For this review, take the finished solid that the model builds, in its own axes (mm). Face numbers are marked on the shaded views. Round coordinates to 2 decimals unless told otherwise and drop trailing zeros. Write each loop counter-clockwise with the first axis right and the second up, starting at its lowest first coordinate (ties: lowest second). Pieces come first, ordered by that corner, then holes. Notation, with made-up numbers: M 6,23 L 20,23 A30 cw 20,56 Z; hole C 63,14.5 d7. An arc over 180 degrees is marked long. Answer in a Markdown table with one row per item.
```python
from build123d import *

# Parameters (mm, degrees)
F0_R     = 14.8209
F0_R_2   = 9.525
F1_DEPTH = 39.116
F2_SIZE2 = 1.524
F2_SIZE  = 1.524
F5_D     = 9.525


with BuildPart() as f1:
    # F0 (on Top) → F1 (new body)
    with BuildSketch(Plane.XY):
        Circle(F0_R)
        Circle(F0_R_2, mode=Mode.SUBTRACT)
    extrude(amount=F1_DEPTH)

    # F2
    f2_edges = [f1.edges().sort_by_distance(p)[0] for p in [
        (-14.8209, 0, 39.116),
    ]]
    chamfer(f2_edges, length=F2_SIZE, length2=F2_SIZE2)

    # F5 (through all)
    with Locations(Plane.XZ.offset(14.8209)):
        with Locations((0, 26.416)):
            Hole(F5_D / 2)


solid = f1.part
```
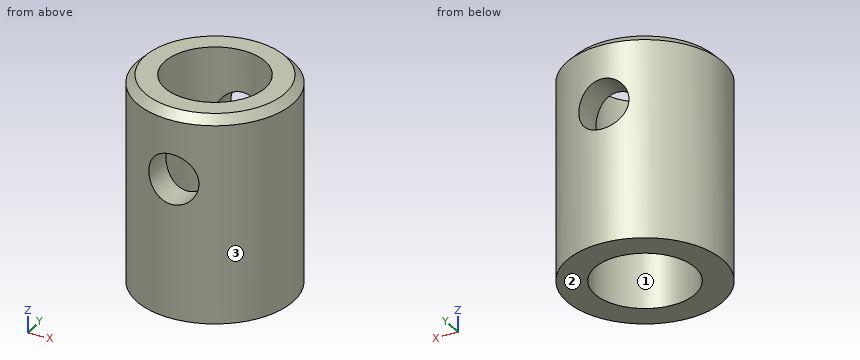
Q1. Take a section at D-D (z = 10). State the section outline as (x, y) points (3 decimals).
Found:
| item | result |
|---|---|
| outline | C 0,0 d29.642; hole C 0,0 d19.05 |
Q2. Take a section at C-C (z = 23). State the section outline as (x, y) points (3 decimals), then the cut area to 3 significant figures.
Found:
| item | result |
|---|---|
| outline | M -3.318,-14.445 L -3.318,-8.928 A9.525 cw -3.318,8.928 L -3.318,14.445 A14.821 ccw Z; M 3.318,-14.445 A14.821 ccw 3.318,14.445 L 3.318,8.928 A9.525 cw 3.318,-8.928 Z |
| area | 334 mm² |
Q3. For probe 1 along Z at (x, y) = (0, 12); probe 2 along Y at (x, z) = (0, 8) (3 decimals); probe 3 along X at (y, z) = (9.5, 23), list the stretches that pass through material, from the lowest coordinate up.
Found:
| item | result |
|---|---|
| probe 1 | 0 to 21.65, 31.18 to 39.12 |
| probe 2 | -14.821 to -9.525, 9.525 to 14.821 |
| probe 3 | -11.38 to -3.32, 3.32 to 11.38 |
Q4. Take a section at B-B (y = 0). State the section outline as (x, z) points (3 decimals).
Found:
| item | result |
|---|---|
| outline | M -14.821,0 L -9.525,0 L -9.525,39.116 L -13.297,39.116 L -14.821,37.592 Z; M 9.525,0 L 14.821,0 L 14.821,37.592 L 13.297,39.116 L 9.525,39.116 Z |
Q5. Take a section at A-A (x = 0). State the section outline as (y, z) points (1 decimal).
Found:
| item | result |
|---|---|
| outline | M -14.8,0 L -9.5,0 L -9.5,21.7 L -14.8,21.7 Z; M -14.8,31.2 L -9.5,31.2 L -9.5,39.1 L -13.3,39.1 L -14.8,37.6 Z; M 9.5,0 L 14.8,0 L 14.8,21.7 L 9.5,21.7 Z; M 9.5,31.2 L 14.8,31.2 L 14.8,37.6 L 13.3,39.1 L 9.5,39.1 Z |
Q6. Mouldability with a two-part tool opening along X and no side actions: class the marked faces 1, 2 and 3 as +X half, -X half, draft (parallel to the pull), parting line (faces both ways), or undercut.
Found:
| item | result |
|---|---|
| face 1 | undercut |
| face 2 | draft |
| face 3 | parting line |
Q7. Insertion check: P1, Ø1.5, axis at x = -8, z = 9, coming from the -Y side; P2, Ø7.5, axis at x = 0, z = 26.416, coming from the -Y side; P3, Ø8, axis at x = 8.5, z = 35, coming from the +Y side; P4, Ø1, axis at x = -6.5, z = 7.5, coming from the +Y side. Each pin has a flat end and moves straight along its axis. Give the tip position at first contact, or say it passes through.
Found:
| item | result |
|---|---|
| P1 | y = -12.93 |
| P2 | through |
| P3 | y = 14.12 |
| P4 | y = 13.55 |
